```python
from build123d import *

# Parameters (mm, degrees)
F0_W     = 101.6
F0_H     = 76.2
F1_DEPTH = 25.4
F2_R     = 19.05
F3_DEPTH = 25.4
F4_R     = 15.24
F5_DEPTH = 76.2


with BuildPart() as f1:
    # F0 (on Front) → F1 (new body)
    with BuildSketch(Plane.XZ):
        Rectangle(F0_W, F0_H)
    extrude(amount=F1_DEPTH)

    # F2 (on face) → F3 (join)
    with BuildSketch(Plane.XZ.offset(25.4)):
        Circle(F2_R)
    extrude(amount=F3_DEPTH)

    # F4 (on face) → F5 (cut)
    with BuildSketch(Plane.XZ.offset(50.8)):
        Circle(F4_R)
    extrude(amount=-F5_DEPTH, mode=Mode.SUBTRACT)


solid = f1.part
```
Can you work these out from the model? Positions are in its coordinate system, mm. A direction names the side the tool comes from. Round coordinates to 2 decimals unless told otherwise and drop trailing zeros. Loops run counter-clockwise (first coordinate to the right, second up) from the corner with the lowest first, then second, coordinate; pieces in that order, holes last. Notation, with made-up numbers: M 55,-30 L 88,-30 A30 ccw 88,3 Z; hole C 66,-7 d10. An arc over 180 degrees is marked long. Write item = value, one per line. Start each with the question number.
(1) Suppose I cut it at B-B on z = 0. Write out the boundary of the cut face in (x, y), plus the area to 3 significant figures.
(2) Suppose I cut it at A-A on x = 0. Write out the boundary of the cut face in (y, z).
(3) I need wall thicknesses on line 1 along Z through (x, y) = (0, -22.5); line 2 along Z through (x, y) = (0, -34); line 3 along Y through (x, z) = (-32.5, -17). Which ranges of each line are inside material? Lowest first, please.
(4) I'm going to push flat-ended pins straight in: P1, Ø5, axis at y = -35.5, z = 12, coming from the -X side; P2, Ø1.5, axis at x = -15, z = -16.5, coming from the -Y side. Where does each tip first touch, or does it pass through?
(5) Suppose I cut it at C-C on y = -24. Write out the boundary of the cut face in (x, z), plus the area to 3 significant figures.
(6) Suppose I cut it at D-D on z = 27.5. Write out the boundary of the cut face in (x, y).
(7) Which directions (+Z, -Z, +X, -X, +Y, -Y) give clear straight access to the entire face, cutting with the end or side of a thin tool? Please do faces 1 (the face through (-3.3, -25.76, -14.88)), 2 (the face through (-15.12, -37.92, -11.59)).
Answer block:
q1.outline = M -50.8,-25.4 L -19.05,-25.4 L -19.05,-50.8 L -15.24,-50.8 L -15.24,0 L -50.8,0 Z; M 15.24,-50.8 L 19.05,-50.8 L 19.05,-25.4 L 50.8,-25.4 L 50.8,0 L 15.24,0 Z
q1.area = 2,000 mm²
q2.outline = M -50.8,-19.05 L -25.4,-19.05 L -25.4,-38.1 L 0,-38.1 L 0,-15.24 L -50.8,-15.24 Z; M -50.8,15.24 L 0,15.24 L 0,38.1 L -25.4,38.1 L -25.4,19.05 L -50.8,19.05 Z
q3.line_1 = -38.1 to -15.24, 15.24 to 38.1
q3.line_2 = -19.05 to -15.24, 15.24 to 19.05
q3.line_3 = -25.4 to 0
q4.P1 = -16.51
q4.P2 = -25.4
q5.outline = M -50.8,-38.1 L 50.8,-38.1 L 50.8,38.1 L -50.8,38.1 Z; hole C 0,0 d30.48
q5.area = 7,010 mm²
q6.outline = M -50.8,-25.4 L 50.8,-25.4 L 50.8,0 L -50.8,0 Z
q7.face_1 = +Y, -Y
q7.face_2 = -Y
